```python
from build123d import *

# Parameters (mm, degrees)
SKETCH1_R      = 3.4
EXTRUDE1_DEPTH = 300


with BuildPart() as part:
    # Sketch1 → Extrude1 (new body)
    with BuildSketch(Plane.XY):
        with BuildLine():
            Line((2.355963526, 7.7), (-2.355963526, 7.7))
            ThreePointArc((-2.355963526, 7.7), (-4.173633293, 8.061556996), (-5.714579315, 9.091184211))
            Line((-5.714579315, 9.091184211), (-10.024617928, 13.401222824))
            ThreePointArc((-10.024617928, 13.401222824), (-10.217328904, 13.689635181), (-10.285, 14.029840753))
            Line((-10.285, 14.029840753), (-10.285, 15.432464473))
            ThreePointArc((-10.285, 15.432464473), (-9.913025612, 16.330490085), (-9.015, 16.702464473))
            Line((-9.015, 16.702464473), (-6.878524829, 16.702464473))
            Line((-6.878524829, 16.702464473), (-6.878524829, 15.94))
            Line((-6.878524829, 15.94), (-5.6348, 15.94))
            ThreePointArc((-5.6348, 15.94), (-4.521248241, 16.401248241), (-4.06, 17.5148))
            Line((-4.06, 17.5148), (-4.06, 18.4252))
            ThreePointArc((-4.06, 18.4252), (-4.521248241, 19.538751759), (-5.6348, 20))
            Line((-5.6348, 20), (-13.185697325, 20))
            Line((-13.185697325, 20), (-16.825, 20))
            ThreePointArc((-16.825, 20), (-19.07006403, 19.07006403), (-20, 16.825))
            Line((-20, 16.825), (-20, -16.825))
            ThreePointArc((-20, -16.825), (-19.07006403, -19.07006403), (-16.825, -20))
            Line((-16.825, -20), (0, -20))
            Line((0, -20), (16.825, -20))
            ThreePointArc((16.825, -20), (19.07006403, -19.07006403), (20, -16.825))
            Line((20, -16.825), (20, -13.049478217))
            Line((20, -13.049478217), (20, -5.6348))
            ThreePointArc((20, -5.6348), (19.538751759, -4.521248241), (18.4252, -4.06))
            Line((18.4252, -4.06), (17.5148, -4.06))
            ThreePointArc((17.5148, -4.06), (16.401248241, -4.521248241), (15.94, -5.6348))
            Line((15.94, -5.6348), (15.94, -6.878524829))
            Line((15.94, -6.878524829), (16.702464473, -6.878524829))
            Line((16.702464473, -6.878524829), (16.702464473, -9.015))
            ThreePointArc((16.702464473, -9.015), (16.330490085, -9.913025612), (15.432464473, -10.285))
            Line((15.432464473, -10.285), (12.495583974, -10.285))
            ThreePointArc((12.495583974, -10.285), (12.155378402, -10.217328904), (11.866966045, -10.024617928))
            Line((11.866966045, -10.024617928), (9.076184211, -7.233836094))
            ThreePointArc((9.076184211, -7.233836094), (8.046556996, -5.692890072), (7.685, -3.875220305))
            Line((7.685, -3.875220305), (7.685, 2.340963526))
            ThreePointArc((7.685, 2.340963526), (8.046556996, 4.158633293), (9.076184211, 5.699579315))
            Line((9.076184211, 5.699579315), (13.401222824, 10.024617928))
            ThreePointArc((13.401222824, 10.024617928), (13.689635181, 10.217328904), (14.029840753, 10.285))
            Line((14.029840753, 10.285), (15.432, 10.285))
            ThreePointArc((15.432, 10.285), (16.330025612, 9.913025612), (16.702, 9.015))
            Line((16.702, 9.015), (16.702, 6.878524829))
            Line((16.702, 6.878524829), (15.94, 6.878524829))
            Line((15.94, 6.878524829), (15.94, 5.6348))
            ThreePointArc((15.94, 5.6348), (16.401248241, 4.521248241), (17.5148, 4.06))
            Line((17.5148, 4.06), (18.4252, 4.06))
            ThreePointArc((18.4252, 4.06), (19.538751759, 4.521248241), (20, 5.6348))
            Line((20, 5.6348), (20, 12.980521783))
            Line((20, 12.980521783), (20, 16.825))
            ThreePointArc((20, 16.825), (19.07006403, 19.07006403), (16.825, 20))
            Line((16.825, 20), (13.070898915, 20))
            Line((13.070898915, 20), (5.6348, 20))
            ThreePointArc((5.6348, 20), (4.521248241, 19.538751759), (4.06, 18.4252))
            Line((4.06, 18.4252), (4.06, 17.5148))
            ThreePointArc((4.06, 17.5148), (4.521248241, 16.401248241), (5.6348, 15.94))
            Line((5.6348, 15.94), (6.878524829, 15.94))
            Line((6.878524829, 15.94), (6.878524829, 16.702464473))
            Line((6.878524829, 16.702464473), (9.015, 16.702464473))
            ThreePointArc((9.015, 16.702464473), (9.913025612, 16.330490085), (10.285, 15.432464473))
            Line((10.285, 15.432464473), (10.285, 14.029840753))
            ThreePointArc((10.285, 14.029840753), (10.217328904, 13.689635181), (10.024617928, 13.401222824))
            Line((10.024617928, 13.401222824), (5.714579315, 9.091184211))
            ThreePointArc((5.714579315, 9.091184211), (4.173633293, 8.061556996), (2.355963526, 7.7))
        make_face()
        Circle(SKETCH1_R, mode=Mode.SUBTRACT)
        with BuildLine():
            Line((-2.291485309, -7.67), (3.30475018, -7.67))
            ThreePointArc((3.30475018, -7.67), (5.122419947, -8.031556996), (6.663365969, -9.061184211))
            Line((6.663365969, -9.061184211), (8.607245789, -11.00506403))
            ThreePointArc((8.607245789, -11.00506403), (9.637289921, -11.693317516), (10.852309819, -11.935))
            Line((10.852309819, -11.935), (17.855103644, -11.935))
            ThreePointArc((17.855103644, -11.935), (18.205048213, -12.079951787), (18.35, -12.429896356))
            Line((18.35, -12.429896356), (18.35, -15.556))
            ThreePointArc((18.35, -15.556), (17.531656347, -17.531656347), (15.556, -18.35))
            Line((15.556, -18.35), (0, -18.35))
            Line((0, -18.35), (-15.414104785, -18.35))
            ThreePointArc((-15.414104785, -18.35), (-15.644649678, -18.195954828), (-15.590556207, -17.924008585))
            Line((-15.590556207, -17.924008585), (-9.805562467, -12.139014844))
            ThreePointArc((-9.805562467, -12.139014844), (-9.558352324, -11.973834194), (-9.266748072, -11.915830212))
            Line((-9.266748072, -11.915830212), (-8.820376291, -11.915829642))
            ThreePointArc((-8.820376291, -11.915829642), (-8.528772039, -11.857825659), (-8.281561897, -11.692645009))
            Line((-8.281561897, -11.692645009), (-5.650101098, -9.061184211))
            ThreePointArc((-5.650101098, -9.061184211), (-4.109155076, -8.031556996), (-2.291485309, -7.67))
        make_face(mode=Mode.SUBTRACT)
        with BuildLine():
            Line((-9.076184211, -5.741552749), (-11.62265199, -8.288020528))
            ThreePointArc((-11.62265199, -8.288020528), (-11.787832613, -8.535230605), (-11.845836623, -8.826834781))
            Line((-11.845836623, -8.826834781), (-11.845837163, -9.196755164))
            ThreePointArc((-11.845837163, -9.196755164), (-11.903841173, -9.488359341), (-12.069021796, -9.735569418))
            Line((-12.069021796, -9.735569418), (-17.924008585, -15.590556207))
            ThreePointArc((-17.924008585, -15.590556207), (-18.195954828, -15.644649678), (-18.35, -15.414104785))
            Line((-18.35, -15.414104785), (-18.35, 15.541))
            ThreePointArc((-18.35, 15.541), (-17.531656347, 17.516656347), (-15.556, 18.335))
            Line((-15.556, 18.335), (-12.316, 18.335))
            ThreePointArc((-12.316, 18.335), (-12.046592316, 18.223407684), (-11.935, 17.954))
            Line((-11.935, 17.954), (-11.935, 9.762593298))
            ThreePointArc((-11.935, 9.762593298), (-11.693317516, 8.5475734), (-11.00506403, 7.517529268))
            Line((-11.00506403, 7.517529268), (-9.076184211, 5.588649448))
            ThreePointArc((-9.076184211, 5.588649448), (-8.046556996, 4.047703426), (-7.685, 2.230033659))
            Line((-7.685, 2.230033659), (-7.685, -2.382936959))
            ThreePointArc((-7.685, -2.382936959), (-8.046556996, -4.200606726), (-9.076184211, -5.741552749))
        make_face(mode=Mode.SUBTRACT)
        with BuildLine():
            Line((18.35, 15.556), (18.35, 12.316))
            ThreePointArc((18.35, 12.316), (18.238407684, 12.046592316), (17.969, 11.935))
            Line((17.969, 11.935), (13.205, 11.935))
            ThreePointArc((13.205, 11.935), (12.306974388, 12.306974388), (11.935, 13.205))
            Line((11.935, 13.205), (11.935, 17.969))
            ThreePointArc((11.935, 17.969), (12.046592316, 18.238407684), (12.316, 18.35))
            Line((12.316, 18.35), (15.556, 18.35))
            ThreePointArc((15.556, 18.35), (17.531656347, 17.531656347), (18.35, 15.556))
        make_face(mode=Mode.SUBTRACT)
    extrude(amount=-EXTRUDE1_DEPTH)


solid = part.part
```
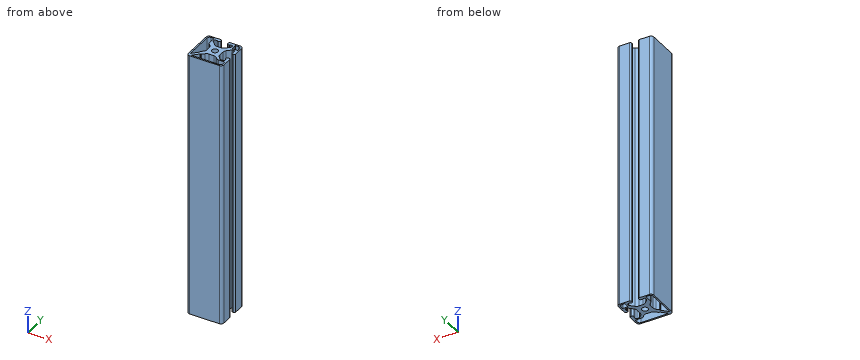
Part model, mm, in its own coordinate system. Round coordinates to 2 decimals unless told otherwise and drop trailing zeros. Use one line per item in the form item = value. Start each with the question number.
Item 1: Band-saw the part on A-A (z = -216.5). Give the number of separate pieces and of enclosed holes in the cut face, plus the area to 3 significant figures.
Item 2: Drop flat-ended pins along their axis: pin 1 Ø2 at (x, z) = (2, -213) entering from +Y; pin 2 Ø0.5 at (x, z) = (18, -89) entering from +Y; pin 3 Ø1 at (x, z) = (18, -168) entering from -Y. Give the stop position or say it passes through.
Item 3: Drill centre lines: line 1 along Y through (x, z) = (0, -116); line 2 along Y through (x, z) = (11, -69.5) (3 decimals); line 3 along X through (y, z) = (-10, -27.5). Where is each one in solid material? Low to high.
Data:
q1.separate_pieces = 1
q1.enclosed_holes = 4
q1.area = 655 mm^2
q2.pin_1 = 7.74
q2.pin_2 = 19.86
q2.pin_3 = -19.93
q3.line_1 = -20 to -18.35, -7.67 to -3.4, 3.4 to 7.7
q3.line_2 = -20 to -18.35, -11.935 to -9.158, 7.623 to 20
q3.line_3 = -20 to -18.35, -12.33 to -6.59, 7.6 to 11.84, 16.23 to 20
